```python
from build123d import *

# Parameters (mm, degrees)
SKETCH1_W           = 50
SKETCH1_H           = 29
BOSS_EXTRUDE1_DEPTH = 5
SKETCH2_W           = 50
SKETCH2_H           = 5
BOSS_EXTRUDE2_DEPTH = 95
SKETCH3_R           = 1.42
CUT_EXTRUDE1_DEPTH  = 60
SKETCH4_R           = 11.1
CUT_EXTRUDE2_DEPTH  = 2.5
SKETCH5_R           = 3.25
CUT_EXTRUDE3_DEPTH  = 10
SKETCH6_R           = 1.75
CUT_EXTRUDE4_DEPTH  = 10
SKETCH8_W           = 2
SKETCH8_H           = 24
BOSS_EXTRUDE3_DEPTH = 32
CUT_EXTRUDE5_DEPTH  = 35
CHAMFER1_SIZE       = 10
FILLET2_R           = 10
FILLET3_R           = 4
FILLET4_R           = 4


with BuildPart() as part:
    # Sketch1 → Boss-Extrude1 (new body)
    with BuildSketch(Plane(origin=(0, 0, 0), x_dir=(1, 0, 0), z_dir=(0, 1, 0))):
        Rectangle(SKETCH1_W, SKETCH1_H)
    extrude(amount=BOSS_EXTRUDE1_DEPTH)

    # Sketch2 → Boss-Extrude2 (add)
    with BuildSketch(Plane(origin=(0, 5, 0), x_dir=(1, 0, 0), z_dir=(0, 1, 0))):
        with Locations((0, 12)):
            Rectangle(SKETCH2_W, SKETCH2_H)
    extrude(amount=BOSS_EXTRUDE2_DEPTH)

    # Sketch3 → Cut-Extrude1 (cut)
    with BuildSketch(Plane.XY.offset(-9.5)):
        with Locations((-15.5, 49)):
            Circle(SKETCH3_R)
        with Locations((15.5, 49)):
            Circle(SKETCH3_R)
        with Locations((15.5, 80)):
            Circle(SKETCH3_R)
        with Locations((-15.5, 80)):
            Circle(SKETCH3_R)
    extrude(amount=-CUT_EXTRUDE1_DEPTH, mode=Mode.SUBTRACT)

    # Sketch4 → Cut-Extrude2 (cut)
    with BuildSketch(Plane.XY.offset(-9.5)):
        with Locations((0, 64.5)):
            Circle(SKETCH4_R)
    extrude(amount=-CUT_EXTRUDE2_DEPTH, mode=Mode.SUBTRACT)

    # Sketch5 → Cut-Extrude3 (cut)
    with BuildSketch(Plane.XY.offset(-12)):
        with Locations((0, 64.5)):
            Circle(SKETCH5_R)
    extrude(amount=-CUT_EXTRUDE3_DEPTH, mode=Mode.SUBTRACT)

    # Sketch6 → Cut-Extrude4 (cut)
    with BuildSketch(Plane(origin=(0, 5, 0), x_dir=(1, 0, 0), z_dir=(0, 1, 0))):
        with Locations(Location((-19, 3.5, 0), (0, 0, 270))):
            Circle(SKETCH6_R)
        with Locations(Location((-19, -8.5, 0), (0, 0, 270))):
            Circle(SKETCH6_R)
        with Locations(Location((19, -8.5, 0), (0, 0, 270))):
            Circle(SKETCH6_R)
        with Locations(Location((19, 3.5, 0), (0, 0, 270))):
            Circle(SKETCH6_R)
    extrude(amount=-CUT_EXTRUDE4_DEPTH, mode=Mode.SUBTRACT)

    # Sketch8 → Boss-Extrude3 (add)
    with BuildSketch(Plane(origin=(0, 5, 0), x_dir=(1, 0, 0), z_dir=(0, 1, 0))):
        with Locations((0, -2.5)):
            Rectangle(SKETCH8_W, SKETCH8_H)
    extrude(amount=BOSS_EXTRUDE3_DEPTH)

    # Sketch9 → Cut-Extrude5 (cut)
    with BuildSketch(Plane(origin=(1, 0, 0), x_dir=(0, 0, -1), z_dir=(1, 0, 0))):
        Polygon((9.5, 37), (-14.5, 5), (-14.5, 37), align=None)
    extrude(amount=-CUT_EXTRUDE5_DEPTH, mode=Mode.SUBTRACT)

    # Chamfer1
    chamfer1_edges = [part.edges().sort_by_distance(p)[0] for p in [
        (-25, 100, -12),
        (25, 100, -12),
    ]]
    chamfer(chamfer1_edges, length=CHAMFER1_SIZE)

    # Fillet2
    fillet2_edges = [part.edges().sort_by_distance(p)[0] for p in [
        (15, 100, -12),
        (-15, 100, -12),
    ]]
    fillet(fillet2_edges, radius=FILLET2_R)

    # Fillet3
    fillet3_edges = [part.edges().sort_by_distance(p)[0] for p in [
        (25, 90, -12),
    ]]
    fillet(fillet3_edges, radius=FILLET3_R)

    # Fillet4
    fillet4_edges = [part.edges().sort_by_distance(p)[0] for p in [
        (-25, 90, -12),
    ]]
    fillet(fillet4_edges, radius=FILLET4_R)


solid = part.part
```
Could you check a few things on this model? Use its own coordinates, in mm. A direction names the side the tool comes from. Coordinates: 2 decimals unless noted, no trailing zeros. Write each loop counter-clockwise with the first axis right and the second up, starting at its lowest first coordinate (ties: lowest second). Pieces come first, ordered by that corner, then holes. Notation, with made-up numbers: (89.25, 88.5) -> (118.25, 88.5) arc R26 cw to (118.25, 114.5) -> close; hole circle Ø11 at (-37, 89). An arc over 180 degrees is marked (long way). Return JSON: item names as keys, results as strings.
(1) Imagine slicing it at C-C, the plane z = 8.5. Please give me the cut outline in (x, y).
Numbers:
{"outline": "(-25, 0) -> (-20.75, 0) -> (-20.75, 5) -> (-25, 5) -> close; (-17.25, 0) -> (17.25, 0) -> (17.25, 5) -> (1, 5) -> (1, 13) -> (-1, 13) -> (-1, 5) -> (-17.25, 5) -> close; (20.75, 0) -> (25, 0) -> (25, 5) -> (20.75, 5) -> close"}
(2) Imagine slicing it at D-D, the plane x = 2. Please give me the cut outline in (y, z), then the cut area to 3 significant figures.
Numbers:
{"outline": "(0, -14.5) -> (61.94, -14.5) -> (61.94, -12) -> (53.58, -12) -> (53.58, -9.5) -> (5, -9.5) -> (5, 14.5) -> (0, 14.5) -> close; (67.06, -14.5) -> (100, -14.5) -> (100, -9.5) -> (75.42, -9.5) -> (75.42, -12) -> (67.06, -12) -> close", "area": "553 mm2"}
(3) I'm going to push flat-ended pins straight in: pin 1 (10 mm diameter, centred on x = 11, y = 86.5, fed in from +Z); pin 2 (8 mm diameter, centred on x = 5.5, z = 1, fed in from +Y); pin 3 (11 mm diameter, centred on x = 4, y = 61.5, fed in from +Z). Where does each tip first touch, or does it pass through?
Numbers:
{"pin 1": "stops at z = -9.5", "pin 2": "stops at y = 5", "pin 3": "stops at z = -12"}
(4) I need wall thicknesses on L1, parallel to X at y = 80, z = -11.65; L2, parallel to Y at x = 0, z = -13.1; L3, parallel to Y at x = 0, z = -10.3. Which ranges of each line are inside material? Lowest first, please.
Numbers:
{"L1": "x = -25 to -16.92, -14.08 to 14.08, 16.92 to 25", "L2": "y = 0 to 61.25, 67.75 to 100", "L3": "y = 0 to 53.4, 75.6 to 100"}
(5) Imagine slicing it at B-B, the plane y = 64.5. Please give me the cut outline in (x, z).
Numbers:
{"outline": "(-25, -14.5) -> (-3.25, -14.5) -> (-3.25, -12) -> (-11.1, -12) -> (-11.1, -9.5) -> (-25, -9.5) -> close; (3.25, -14.5) -> (25, -14.5) -> (25, -9.5) -> (11.1, -9.5) -> (11.1, -12) -> (3.25, -12) -> close"}
(6) Which directions (+Z, -Z, +X, -X, +Y, -Y) give clear straight access to the entire face, cutting with the end or side of a thin tool? Please do faces 1 (the flat face through (-1, 14, -3)), 2 (the cylindrical face through (-24.69, 89.89, -12.04)), 3 (the flat face through (1, 14, -3)).
Numbers:
{"face 1": "+Z, -X, +Y", "face 2": "+Z, -Z, -X, +Y", "face 3": "+Z, +X, +Y"}
(7) We'd pull the mould along Z, two halves only. Please class faces 4 (the cylindrical face through (-17.265, 2.535, -3.728)), 5 (the flat face through (2.3, 67.1, -12)), 6 (the flat face through (-21, 94, -12)): +Z half, -Z half, draft (parallel to the pull), parting line (faces both ways), or undercut.
Numbers:
{"face 4": "undercut", "face 5": "+Z half", "face 6": "draft"}
(8) Imagine slicing it at A-A, the plane x = 19. Please give me the cut outline in (y, z).
Numbers:
{"outline": "(0, -14.5) -> (96, -14.5) -> (96, -9.5) -> (5, -9.5) -> (5, -5.25) -> (0, -5.25) -> close; (0, -1.75) -> (5, -1.75) -> (5, 6.75) -> (0, 6.75) -> close; (0, 10.25) -> (5, 10.25) -> (5, 14.5) -> (0, 14.5) -> close"}
